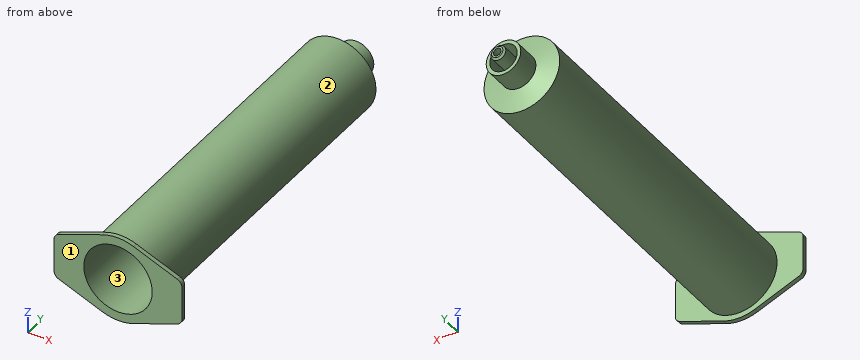
```python
from build123d import *

# Parameters (mm, degrees)
SKETCH_2_R      = 9.5
EXTRUDE_1_DEPTH = 1.2


with BuildPart() as part:
    # Эскиз1 → Повернуть1 (revolve)
    with BuildSketch(Plane.XY, mode=Mode.PRIVATE) as revolve_1_sk:
        Polygon((1.05, 5.570639193), (1.55, 5.570639193), (2.05, 5.070639193), (2.05, -3.008676838), (3.8, -3.447871743), (3.8, 2.870639193), (4.8, 2.870639193), (4.8, -3.69884026), (10.5, -5.129360807), (10.5, -99.629360807), (9.5, -99.629360807), (9.5, -5.909404025), (1.05, -3.788720055), align=None)
    revolve(revolve_1_sk.sketch.rotate(Axis((0, 0, 0), (0, -1, 0)), 90), axis=Axis((0, 0, 0), (0, -1, 0)))

    # Эскиз2 → Бобышка-Вытянуть1 (add)
    with BuildSketch(Plane.XZ.offset(99.629360807)):
        with BuildLine():
            Line((16.471592317, -6.494555517), (4.329553903, -11.191736371))
            ThreePointArc((4.329553903, -11.191736371), (0, -12), (-4.329553903, -11.191736371))
            Line((-4.329553903, -11.191736371), (-16.471592317, -6.494555517))
            ThreePointArc((-16.471592317, -6.494555517), (-17.399724922, -5.759933042), (-17.75, -4.629266122))
            Line((-17.75, -4.629266122), (-17.75, 4.629266122))
            ThreePointArc((-17.75, 4.629266122), (-17.399724922, 5.759933042), (-16.471592317, 6.494555517))
            Line((-16.471592317, 6.494555517), (-4.329553903, 11.191736371))
            ThreePointArc((-4.329553903, 11.191736371), (0, 12), (4.329553903, 11.191736371))
            Line((4.329553903, 11.191736371), (16.471592317, 6.494555517))
            ThreePointArc((16.471592317, 6.494555517), (17.399724922, 5.759933042), (17.75, 4.629266122))
            Line((17.75, 4.629266122), (17.75, -4.629266122))
            ThreePointArc((17.75, -4.629266122), (17.399724922, -5.759933042), (16.471592317, -6.494555517))
        make_face()
        with Locations(Location((0, 0, 0), (0, 0, 270))):
            Circle(SKETCH_2_R, mode=Mode.SUBTRACT)
    extrude(amount=EXTRUDE_1_DEPTH)


solid = part.part
```
Could you check a few things on this model? Use its own coordinates, in mm. Face numbers are marked on the shaded views. A direction names the side the tool comes from. Round coordinates to 2 decimals unless told otherwise and drop trailing zeros. Write each loop counter-clockwise with the first axis right and the second up, starting at its lowest first coordinate (ties: lowest second). Pieces come first, ordered by that corner, then holes. Notation, with made-up numbers: M 49.5,32.25 L 101.5,32.25 A21 ccw 101.5,67.25 Z; hole C 75.5,62.25 d10. An arc over 180 degrees is marked long. Write each question's results on one line, items separated by ' | '. Start each with the question number.
1. I need wall thicknesses on L1, parallel to X at y = -1.75, z = 0; L2, parallel to X at y = -48, z = 0; L3, parallel to Y at x = -14.5, z = 4.5. Which ranges of each line are inside material? Lowest first, please. Write a range as from..to.
2. Imagine slicing it at B-B on y = -15.5. List the corners of the cut face in (x, z) for me.
3. Imagine slicing it at C-C on x = -12.5. List the corners of the cut face in (y, z) for me.
4. I'm going to push flat-ended pins straight in: pin 1 Ø4 at (x, z) = (2.5, 7.5) entering from +Y; pin 2 Ø11.5 at (x, z) = (0, 0) entering from +Y; pin 3 Ø5 at (x, y) = (9.5, -76) entering from +Z; pin 4 Ø1.5 at (y, z) = (-21, -4) entering from +X. Where does each tip first touch, or does it pass through?
5. On a 3-axis mill with a long thin cutter (end or side, diameter ignored), from which of +Z, -Z, +X, -X, +Y, -Y can I reach the whole of each face in a straight line? I mean the marked faces 1, 2 and 3. Say none if no direction works.
Result sheet:
1) L1: x = -4.8..-3.8, -2.05..-1.05, 1.05..2.05, 3.8..4.8 | L2: x = -10.5..-9.5, 9.5..10.5 | L3: y = -100.83..-99.63
2) outline: C 0,0 d21; hole C 0,0 d19
3) outline: M -100.83,-8.03 L -99.63,-8.03 L -99.63,8.03 L -100.83,8.03 Z
4) pin 1: stops at y = -3.98 | pin 2: stops at y = 5.57 | pin 3: stops at z = 7.83 | pin 4: stops at x = 9.98
5) face 1: +Z, -Z, +X, -X, -Y | face 2: +Y | face 3: -Y
